Verification items for the finished model (mm, model axes). A direction names the side the tool comes from. Round coordinates to 2 decimals unless told otherwise and drop trailing zeros. Write each loop counter-clockwise with the first axis right and the second up, starting at its lowest first coordinate (ties: lowest second). Pieces come first, ordered by that corner, then holes. Notation, with made-up numbers: (83, 63) - (130, 63) arc R28 cw to (130, 97) - close; hole circle Ø4 at (-5.5, -17.75). An arc over 180 degrees is marked (long way). Answer as a JSON object with one key per item and string values.
```python
from build123d import *

# Parameters (mm, degrees)
BOSS_EXTRUDE1_DEPTH     = 2
BOSS_EXTRUDE2_DEPTH     = 11
CUT_EXTRUDE1_DEPTH      = 11
CUT_EXTRUDE1_DEPTH_BACK = 11


with BuildPart() as part:
    # Sketch1 → Boss-Extrude1 (new body)
    # profile 1 of 7: a face of its own
    with BuildSketch(Plane(origin=(0, 0, 0), x_dir=(1, 0, 0), z_dir=(0, 1, 0))):
        Polygon((-22.03308425, 10.5), (-40, 10.5), (-40, 5.5), (-34, 5.5), (-34, 4.5), (-40, 4.5), (-40, 3.5), (-34, 3.5), (-34, 2.5), (-40, 2.5), (-40, -8.5), (-14, -8.5), (-14, 3.5), (-8, 3.5), (-8, 4.5), (-14.03308425, 4.5), (-14.03308425, 8.5), (-22.03308425, 8.5), align=None)
    # profile 2 of 7: a face of its own
    with BuildSketch(Plane(origin=(0, 0, 0), x_dir=(1, 0, 0), z_dir=(0, 1, 0))):
        Polygon((-40, 10.5), (-42, 10.5), (-42, -10.5), (-6, -10.5), (40, -5), (40, 5), (-6, 10.5), (-22.03308425, 10.5), (-22.03308425, 8.5), (-14.03308425, 8.5), (-14.03308425, 4.5), (-8, 4.5), (-8, 3.5), (-14, 3.5), (-14, -8.5), (-40, -8.5), (-40, 2.5), (-34, 2.5), (-34, 3.5), (-40, 3.5), (-40, 4.5), (-34, 4.5), (-34, 5.5), (-40, 5.5), align=None)
        Polygon((-6, -8.5), (-6, 8.5), (-2, 8.02044412), (2, 7.540888241), (32, 3.944219144), (34, 3.704441204), (38, 3.224885324), (38, -3.224885324), (34, -3.704441204), (32, -3.944219144), (2, -7.540888241), (-2, -8.02044412), align=None, mode=Mode.SUBTRACT)
    # profile 3 of 7: a face of its own
    with BuildSketch(Plane(origin=(0, 0, 0), x_dir=(1, 0, 0), z_dir=(0, 1, 0))):
        Polygon((2, 7.540888241), (-2, 8.02044412), (-2, 4.02044412), (2, 4.02044412), align=None)
    # profile 4 of 7: a face of its own
    with BuildSketch(Plane(origin=(0, 0, 0), x_dir=(1, 0, 0), z_dir=(0, 1, 0))):
        Polygon((-2, 8.02044412), (-6, 8.5), (-6, -8.5), (-2, -8.02044412), (-2, -4.02044412), (2, -4.02044412), (2, -7.540888241), (32, -3.944219144), (32, 3.944219144), (2, 7.540888241), (2, 4.02044412), (-2, 4.02044412), align=None)
    # profile 5 of 7: a face of its own
    with BuildSketch(Plane(origin=(0, 0, 0), x_dir=(1, 0, 0), z_dir=(0, 1, 0))):
        Polygon((34, 3.704441204), (32, 3.944219144), (32, -3.944219144), (34, -3.704441204), align=None)
    # profile 6 of 7: a face of its own
    with BuildSketch(Plane(origin=(0, 0, 0), x_dir=(1, 0, 0), z_dir=(0, 1, 0))):
        Polygon((-2, -4.02044412), (-2, -8.02044412), (2, -7.540888241), (2, -4.02044412), align=None)
    # profile 7 of 7: a face of its own
    with BuildSketch(Plane(origin=(0, 0, 0), x_dir=(1, 0, 0), z_dir=(0, 1, 0))):
        Polygon((38, 3.224885324), (34, 3.704441204), (34, -3.704441204), (38, -3.224885324), align=None)
    extrude(amount=BOSS_EXTRUDE1_DEPTH)

    # Sketch1_5 → Boss-Extrude2 (add)
    # profile 1 of 4: a face of its own
    with BuildSketch(Plane(origin=(0, 0, 0), x_dir=(1, 0, 0), z_dir=(0, 1, 0))):
        Polygon((-40, 10.5), (-42, 10.5), (-42, -10.5), (-6, -10.5), (40, -5), (40, 5), (-6, 10.5), (-22.03308425, 10.5), (-22.03308425, 8.5), (-14.03308425, 8.5), (-14.03308425, 4.5), (-8, 4.5), (-8, 3.5), (-14, 3.5), (-14, -8.5), (-40, -8.5), (-40, 2.5), (-34, 2.5), (-34, 3.5), (-40, 3.5), (-40, 4.5), (-34, 4.5), (-34, 5.5), (-40, 5.5), align=None)
        Polygon((-6, -8.5), (-6, 8.5), (-2, 8.02044412), (2, 7.540888241), (32, 3.944219144), (34, 3.704441204), (38, 3.224885324), (38, -3.224885324), (34, -3.704441204), (32, -3.944219144), (2, -7.540888241), (-2, -8.02044412), align=None, mode=Mode.SUBTRACT)
    # profile 2 of 4: a face of its own
    with BuildSketch(Plane(origin=(0, 0, 0), x_dir=(1, 0, 0), z_dir=(0, 1, 0))):
        Polygon((2, 7.540888241), (-2, 8.02044412), (-2, 4.02044412), (2, 4.02044412), align=None)
    # profile 3 of 4: a face of its own
    with BuildSketch(Plane(origin=(0, 0, 0), x_dir=(1, 0, 0), z_dir=(0, 1, 0))):
        Polygon((-2, -4.02044412), (-2, -8.02044412), (2, -7.540888241), (2, -4.02044412), align=None)
    # profile 4 of 4: a face of its own
    with BuildSketch(Plane(origin=(0, 0, 0), x_dir=(1, 0, 0), z_dir=(0, 1, 0))):
        Polygon((34, 3.704441204), (32, 3.944219144), (32, -3.944219144), (34, -3.704441204), align=None)
    extrude(amount=BOSS_EXTRUDE2_DEPTH)

    # Sketch2 → Cut-Extrude1 (cut, two sides: drawn at the far end of the back side and taken through both)
    with BuildSketch(Plane.XY.offset(-CUT_EXTRUDE1_DEPTH_BACK)):
        Polygon((-6, 11), (40, 11), (40, 8), align=None)
    extrude(amount=CUT_EXTRUDE1_DEPTH + CUT_EXTRUDE1_DEPTH_BACK, mode=Mode.SUBTRACT)


solid = part.part
```
Q1. Section check D-D, the plane z = 6.25. Record the cut outline in (x, y), then the cut area to 3 significant figures.
Geometry check:
{"outline": "(-42, 0) - (29.55, 0) - (29.55, 8.68) - (12.77, 9.78) - (12.77, 2) - (2, 2) - (2, 10.48) - (-2, 10.74) - (-2, 2) - (-6, 2) - (-6, 11) - (-14, 11) - (-14, 2) - (-40, 2) - (-40, 11) - (-42, 11) - close", "area": "389 mm2"}
Q2. Set-up check for faces 1 (the flat face through (-37, 6, -5.5)), 2 (the flat face through (17.32, 4.2, -7.71)), 3 (the flat face through (-40, 6, 3)): record each of +Z, -Z, +X, -X, +Y, -Y from which the full face is reachable in a straight line by a thin tool's end or side.
Geometry check:
{"face 1": "-Z, +Y", "face 2": "-Z, +X, +Y, -Y", "face 3": "+Y"}
Q3. Release check for a two-part mould opening along X. For faces 4 (the flat face through (-20, 11, 9)), 5 (the flat face through (-4.028, 6.437, -8.264)), 6 (the flat face through (40, 4, 0)), 7 (the flat face through (-2, 6, 6)) record: released by +X, released by -X, zero draft, split by the parting line, or undercut.
Geometry check:
{"face 4": "zero draft", "face 5": "undercut", "face 6": "released by +X", "face 7": "undercut"}
Q4. Gauge pin test, flat ends, axial feed: P1, Ø6, axis at x = 29.5, z = 2, coming from the +Y side; P2, Ø3, axis at x = 0, y = 7.5, coming from the +Z side; P3, Ø5, axis at x = 7.5, y = 9, coming from the -Z side. Record the tip position at first contact, or that the pin passes through.
Geometry check:
{"P1": "stops at y = 8.8", "P2": "stops at z = 9.96", "P3": "stops at z = -9.18"}
Q5. Section check B-B, the plane y = 6. State how many separate pieces and enclosed holes the cut face has, then the cut area to 3 significant figures.
Geometry check:
{"separate pieces": "1", "enclosed holes": "2", "area": "527 mm2"}
Q6. Section check A-A, the plane z = -1.75. Record the cut outline in (x, y).
Geometry check:
{"outline": "(-42, 0) - (40, 0) - (40, 8) - (38, 8.13) - (38, 2) - (34, 2) - (34, 8.39) - (32, 8.52) - (32, 2) - (-6, 2) - (-6, 11) - (-14, 11) - (-14, 2) - (-40, 2) - (-40, 11) - (-42, 11) - close"}
Q7. Material ranges on line 1 along X through (y, z) = (7, 2.5); line 2 along X through (y, z) = (9, 3); line 3 along Z through (x, y) = (-17.5, 10.5), recorded low to high. Write a range as [from, to].
Geometry check:
{"line 1": "x = [-42, -40], [-14, -6], [32, 34], [38, 40]", "line 2": "x = [-42, -40], [-14, -6]", "line 3": "z = [-10.5, -8.5], [8.5, 10.5]"}
Q8. Section check C-C, the plane x = -25. Record the cut outline in (y, z), then the cut area to 3 significant figures.
Geometry check:
{"outline": "(0, -10.5) - (2, -10.5) - (2, 8.5) - (11, 8.5) - (11, 10.5) - (0, 10.5) - close", "area": "60.0 mm2"}
